from build123d import *

# Parameters (mm, degrees)
SKETCH1_R           = 8.7376
BOSS_EXTRUDE1_DEPTH = 12.7
BOSS_EXTRUDE3_DEPTH = 4.516000112
FILLET2_R           = 5
CUT_EXTRUDE10_DEPTH = 12.192
SKETCH23_R          = 1.5875
CUT_EXTRUDE11_DEPTH = 38.364220181
CUT_EXTRUDE13_START = -1.27
SKETCH24_R          = 3.175
SKETCH24_R_2        = 1.5875
CUT_EXTRUDE13_DEPTH = 1.27
FILLET11_R          = 1.778


with BuildPart() as part:
    # Sketch1 → Boss-Extrude1 (new body)
    with BuildSketch(Plane.YZ):
        with Locations(Location((0, 0, 0), (0, 0, 270))):
            Circle(SKETCH1_R)
    extrude(amount=BOSS_EXTRUDE1_DEPTH)

    # Sketch10 → Boss-Extrude3 (add)
    with BuildSketch(Plane(origin=(0, 0, 0), x_dir=(0, -1, 0), z_dir=(-1, 0, 0))):
        with BuildLine():
            Line((0, 8.7376), (34.036, 8.7376))
            Line((34.036, 8.7376), (34.036, -8.7376))
            Line((34.036, -8.7376), (0, -8.7376))
            ThreePointArc((0, -8.7376), (8.7376, 0), (0, 8.7376))
        make_face()
    extrude(amount=-BOSS_EXTRUDE3_DEPTH)

    # Fillet2
    fillet2_edges = [part.edges().sort_by_distance(p)[0] for p in [
        (2.258000056, -34.036, 8.7376),
        (2.258000056, -34.036, -8.7376),
    ]]
    fillet(fillet2_edges, radius=FILLET2_R)

    # Sketch22 → Cut-Extrude10 (cut)
    with BuildSketch(Plane.YZ.offset(12.7)):
        with BuildLine():
            Line((-4.089715516, -2.794), (4.089715516, -2.794))
            ThreePointArc((4.089715516, -2.794), (4.953, 0), (4.089715516, 2.794))
            Line((4.089715516, 2.794), (-4.089715516, 2.794))
            ThreePointArc((-4.089715516, 2.794), (-4.953, 0), (-4.089715516, -2.794))
        make_face()
    extrude(amount=-CUT_EXTRUDE10_DEPTH, mode=Mode.SUBTRACT)

    # Sketch23 → Cut-Extrude11 (cut, through all)
    with BuildSketch(Plane.ZY):
        with Locations((0, -30.089710358)):
            Circle(SKETCH23_R)
        with Locations((0, -20.184348406)):
            Circle(SKETCH23_R)
    extrude(amount=-CUT_EXTRUDE11_DEPTH, mode=Mode.SUBTRACT)

    # Sketch24 → Cut-Extrude13 (cut)
    # profile 1 of 2: a face of its own
    with BuildSketch(Plane.YZ.offset(4.516000112).offset(CUT_EXTRUDE13_START)):
        with Locations(Location((-20.184348406, 0, 0), (0, 0, 270))):
            Circle(SKETCH24_R)
        with Locations(Location((-20.184348406, 0, 0), (0, 0, 90))):
            Circle(SKETCH24_R_2, mode=Mode.SUBTRACT)
    # profile 2 of 2: a face of its own
    with BuildSketch(Plane.YZ.offset(4.516000112).offset(CUT_EXTRUDE13_START)):
        with Locations(Location((-30.089710358, 0, 0), (0, 0, 270))):
            Circle(SKETCH24_R)
    extrude(amount=CUT_EXTRUDE13_DEPTH, mode=Mode.SUBTRACT)

    # Fillet11
    fillet11_edges = [part.edges().sort_by_distance(p)[0] for p in [
        (6.604, 4.089715516, 2.794),
        (6.604, 4.089715516, -2.794),
        (6.604, -4.089715516, -2.794),
        (6.604, -4.089715516, 2.794),
    ]]
    fillet(fillet11_edges, radius=FILLET11_R)


solid = part.part
Geometry: final body of the model. Coordinates: model frame, mm. A direction names the side the tool comes from. Give positions to 0.01 mm unless a question says otherwise; leave off trailing zeros. Loops run counter-clockwise (first coordinate to the right, second up) from the corner with the lowest first, then second, coordinate; pieces in that order, holes last. Notation, with made-up numbers: (20, 1) - (58, 1) arc R26 ccw to (58, 27) - close; hole circle Ø4 at (-23, -7.5). An arc over 180 degrees is marked (long way). One line per question, with ' | ' between items. Start each with the question number.
(1) Ray query, line 1 (Y direction, x = 1.5, z = -1); line 2 (X direction, y = -25.5, z = 4.5); line 3 (Y direction, x = 4.75, z = -2). Return the intervals inside material, ascending. Write a range as from..to.
(2) Section query A-A on x = 10.5. Return loops of the section in (y, z), then the cut area to 3 significant figures.
(3) Section query C-C on y = -29.5. Return loops of the section in (x, z), then the cut area to 3 significant figures.
(4) Reachability of faces 1 (the cylindrical face through (7.672, 8.663, 1.137)), 2 (the flat face through (0, -13, 0)) from +Z, -Z, +X, -X, +Y, -Y: full face, straight path, thin tool, end or side. Return the list, or none.
(5) Section query D-D on x = 3.75. Return loops of the section in (y, z) (3 decimals), then the cut area to 3 significant figures.
(6) Pull-direction query (Z, two-part tool) for faces 3 (the cylindrical face through (2.29, -32.532, 7.312)), 4 (the flat face through (4.516, -17, 2)), 5 (the flat face through (7, 0, 2.794)); classes: released by +Z, released by -Z, zero draft, split by the parting line, or undercut.
(7) Contact query for flat-ended pins moving along their axis: pin 1 (3 mm diameter, centred on y = -19.5, z = 0.5, fed in from +X); pin 2 (8.5 mm diameter, centred on y = -20.18, z = 0, fed in from +X); pin 3 (3 mm diameter, centred on x = 11, y = -7, fed in from -Z). Output: stop coordinate, or through.
(8) Section query B-B on z = 0. Return loops of the section in (x, y).
The answers:
1) line 1: -34.04..-31.32, -28.86..-21.42, -18.95..-4.85, 4.85..8.68 | line 2: 0..4.52 | line 3: -8.51..-4.49, 4.49..8.51
2) outline: circle Ø17.48 at (0, 0); hole (-4.69, -1.58) arc R1.78 ccw to (-3.01, -2.79) - (3.01, -2.79) arc R1.78 ccw to (4.69, -1.58) arc R4.95 ccw to (4.69, 1.58) arc R1.78 ccw to (3.01, 2.79) - (-3.01, 2.79) arc R1.78 ccw to (-4.69, 1.58) arc R4.95 ccw to start | area: 188 mm2
3) outline: (0, -8.72) - (4.52, -8.72) - (4.52, -3.12) - (3.25, -3.12) - (3.25, -1.47) - (0, -1.47) - close; (0, 1.47) - (3.25, 1.47) - (3.25, 3.12) - (4.52, 3.12) - (4.52, 8.72) - (0, 8.72) - close | area: 61.2 mm2
4) face 1: +X | face 2: +Z, -Z, -X, +Y, -Y
5) outline: (-34.036, -3.738) arc R5 ccw to (-29.036, -8.738) - (0, -8.738) arc R8.738 ccw to (0, 8.738) - (-29.036, 8.738) arc R5 ccw to (-34.036, 3.738) - close; hole circle Ø6.35 at (-30.09, 0); hole circle Ø6.35 at (-20.184, 0); hole (-4.693, -1.585) arc R1.778 ccw to (-3.008, -2.794) - (3.008, -2.794) arc R1.778 ccw to (4.693, -1.585) arc R4.953 ccw to (4.693, 1.585) arc R1.778 ccw to (3.008, 2.794) - (-3.008, 2.794) arc R1.778 ccw to (-4.693, 1.585) arc R4.953 ccw to start | area: 589 mm2
6) face 3: released by +Z | face 4: zero draft | face 5: undercut
7) pin 1: x = 3.25 | pin 2: x = 4.52 | pin 3: z = -6.79
8) outline: (0, -34.04) - (4.52, -34.04) - (4.52, -33.26) - (3.25, -33.26) - (3.25, -31.68) - (0, -31.68) - close; (0, -28.5) - (3.25, -28.5) - (3.25, -26.91) - (4.52, -26.91) - (4.52, -23.36) - (3.25, -23.36) - (3.25, -21.77) - (0, -21.77) - close; (0, -18.6) - (3.25, -18.6) - (3.25, -17.01) - (4.52, -17.01) - (4.52, -8.74) - (12.7, -8.74) - (12.7, -4.95) - (0.51, -4.95) - (0.51, 4.95) - (12.7, 4.95) - (12.7, 8.74) - (0, 8.74) - close
